Build history of the part. All positions in model axes, mm. A direction names the side the tool comes from. Give positions to 0.01 mm unless a question says otherwise; leave off trailing zeros. Loops run counter-clockwise (first coordinate to the right, second up) from the corner with the lowest first, then second, coordinate; pieces in that order, holes last. Notation, with made-up numbers: M 38,7 L 80,7 A24 ccw 80,33 Z; hole C 53,57.5 d8. An arc over 180 degrees is marked long. Answer in a Markdown table with one row per item. Add a question column.
```python
from build123d import *

# Parameters (mm, degrees)
F0_W          = 120
F0_H          = 13
F0_R          = 1.5
F1_DEPTH      = 13
F2_W          = 120
F2_H          = 5
F3_DEPTH      = 8
F3_DEPTH_BACK = 8
F4_R          = 2.1741492727
F5_DEPTH      = 13
F6_R          = 2
F7_T1_DEPTH   = 16.5
F7_T3_DEPTH   = 16.5
F7_T6_ANGLE   = 90
F7_T8_ANGLE   = 90
F7_T10_ANGLE  = 90
F7_T12_ANGLE  = 90
F7_T14_ANGLE  = 90
F7_T16_ANGLE  = 90
F7_T18_ANGLE  = 90
F7_T20_ANGLE  = 90


# Not quite as in the source:
# - a fillet or chamfer that OpenCascade refuses, or shapes differently, is made with other operations: its cross-section is extruded or revolved along the edge and cut away or added


with BuildPart() as f1:
    # F0 (on Top) → F1 (new body)
    with BuildSketch(Plane.XY):
        Rectangle(F0_W, F0_H)
        with Locations((-55.5, 0)):
            Circle(F0_R, mode=Mode.SUBTRACT)
    extrude(amount=F1_DEPTH)

    # F2 (on Front) → F3 (cut, two sides)
    with BuildSketch(Plane.XZ) as f3_sk:
        with Locations((0, 6.5)):
            Rectangle(F2_W, F2_H)
    extrude(amount=-F3_DEPTH, mode=Mode.SUBTRACT)
    extrude(f3_sk.sketch, amount=F3_DEPTH_BACK, mode=Mode.SUBTRACT)

    # F4 (on Top) → F5 (join)
    with BuildSketch(Plane.XY):
        with Locations((55.0134144723, 0)):
            Circle(F4_R)
    extrude(amount=F5_DEPTH)

    # F6
    f6_edges = [f1.edges().sort_by_distance(p)[0] for p in [
        (0, -6.5, 13),
        (-60, 0, 13),
        (0, 6.5, 13),
        (60, 0, 13),
        (-60, 0, 0),
        (0, -6.5, 0),
        (60, 0, 0),
        (0, 6.5, 0),
    ]]
    fillet(f6_edges, radius=F6_R)

    # F7: fillet of radius 5 on 8 edges, made by hand

    # F7_s2 → F7_t1 (cut)
    with BuildSketch(Plane.XY.offset(-3.5)):
        with BuildLine():
            ThreePointArc((-55, -6.5), (-58.5355339059, -5.0355339059), (-60, -1.5))
            Line((-60, -1.5), (-60, -6.5))
            Line((-60, -6.5), (-55, -6.5))
        make_face()
        with BuildLine():
            ThreePointArc((-55, 6.5), (-58.5355339059, 5.0355339059), (-60, 1.5))
            Line((-60, 1.5), (-60, 6.5))
            Line((-60, 6.5), (-55, 6.5))
        make_face()
        with BuildLine():
            ThreePointArc((60, -1.5), (58.5355339059, -5.0355339059), (55, -6.5))
            Line((55, -6.5), (60, -6.5))
            Line((60, -6.5), (60, -1.5))
        make_face()
        with BuildLine():
            ThreePointArc((60, 1.5), (58.5355339059, 5.0355339059), (55, 6.5))
            Line((55, 6.5), (60, 6.5))
            Line((60, 6.5), (60, 1.5))
        make_face()
    extrude(amount=F7_T1_DEPTH, mode=Mode.SUBTRACT)

    # F7_s4 → F7_t3 (cut)
    with BuildSketch(Plane.XY):
        with BuildLine():
            ThreePointArc((-55, -6.5), (-58.5355339059, -5.0355339059), (-60, -1.5))
            Line((-60, -1.5), (-60, -6.5))
            Line((-60, -6.5), (-55, -6.5))
        make_face()
        with BuildLine():
            ThreePointArc((-55, 6.5), (-58.5355339059, 5.0355339059), (-60, 1.5))
            Line((-60, 1.5), (-60, 6.5))
            Line((-60, 6.5), (-55, 6.5))
        make_face()
        with BuildLine():
            ThreePointArc((60, -1.5), (58.5355339059, -5.0355339059), (55, -6.5))
            Line((55, -6.5), (60, -6.5))
            Line((60, -6.5), (60, -1.5))
        make_face()
        with BuildLine():
            ThreePointArc((60, 1.5), (58.5355339059, 5.0355339059), (55, 6.5))
            Line((55, 6.5), (60, 6.5))
            Line((60, 6.5), (60, 1.5))
        make_face()
    extrude(amount=F7_T3_DEPTH, mode=Mode.SUBTRACT)

    # F7_s5 → F7_t6 (revolve, cut)
    with BuildSketch(Plane.YZ.offset(55)):
        with BuildLine():
            ThreePointArc((4.5, 0), (5.9142135624, 0.5857864376), (6.5, 2))
            Line((6.5, 2), (6.5, 0))
            Line((6.5, 0), (4.5, 0))
        make_face()
    revolve(axis=Axis((55, 1.5, 0), (0, 0, -1)), revolution_arc=F7_T6_ANGLE, mode=Mode.SUBTRACT)

    # F7_s7 → F7_t8 (revolve, cut)
    with BuildSketch(Plane.XZ.offset(1.5)):
        with BuildLine():
            ThreePointArc((58, 0), (59.4142135624, 0.5857864376), (60, 2))
            Line((60, 2), (60, 0))
            Line((60, 0), (58, 0))
        make_face()
    revolve(axis=Axis((55, -1.5, 0), (0, 0, -1)), revolution_arc=F7_T8_ANGLE, mode=Mode.SUBTRACT)

    # F7_s9 → F7_t10 (revolve, cut)
    with BuildSketch(Plane.XZ.offset(-1.5)):
        with BuildLine():
            ThreePointArc((58, 13), (59.4142135624, 12.4142135624), (60, 11))
            Line((60, 11), (60, 13))
            Line((60, 13), (58, 13))
        make_face()
    revolve(axis=Axis((55, 1.5, 13), (0, 0, 1)), revolution_arc=F7_T10_ANGLE, mode=Mode.SUBTRACT)

    # F7_s11 → F7_t12 (revolve, cut)
    with BuildSketch(Plane.YZ.offset(55)):
        with BuildLine():
            ThreePointArc((-4.5, 13), (-5.9142135624, 12.4142135624), (-6.5, 11))
            Line((-6.5, 11), (-6.5, 13))
            Line((-6.5, 13), (-4.5, 13))
        make_face()
    revolve(axis=Axis((55, -1.5, 13), (0, 0, 1)), revolution_arc=F7_T12_ANGLE, mode=Mode.SUBTRACT)

    # F7_s13 → F7_t14 (revolve, cut)
    with BuildSketch(Plane.XZ.offset(-1.5)):
        with BuildLine():
            ThreePointArc((-58, 0), (-59.4142135624, 0.5857864376), (-60, 2))
            Line((-60, 2), (-60, 0))
            Line((-60, 0), (-58, 0))
        make_face()
    revolve(axis=Axis((-55, 1.5, 0), (0, 0, -1)), revolution_arc=F7_T14_ANGLE, mode=Mode.SUBTRACT)

    # F7_s15 → F7_t16 (revolve, cut)
    with BuildSketch(Plane.YZ.offset(-55)):
        with BuildLine():
            ThreePointArc((-4.5, 0), (-5.9142135624, 0.5857864376), (-6.5, 2))
            Line((-6.5, 2), (-6.5, 0))
            Line((-6.5, 0), (-4.5, 0))
        make_face()
    revolve(axis=Axis((-55, -1.5, 0), (0, 0, -1)), revolution_arc=F7_T16_ANGLE, mode=Mode.SUBTRACT)

    # F7_s17 → F7_t18 (revolve, cut)
    with BuildSketch(Plane.YZ.offset(-55)):
        with BuildLine():
            ThreePointArc((4.5, 13), (5.9142135624, 12.4142135624), (6.5, 11))
            Line((6.5, 11), (6.5, 13))
            Line((6.5, 13), (4.5, 13))
        make_face()
    revolve(axis=Axis((-55, 1.5, 13), (0, 0, 1)), revolution_arc=F7_T18_ANGLE, mode=Mode.SUBTRACT)

    # F7_s19 → F7_t20 (revolve, cut)
    with BuildSketch(Plane.XZ.offset(1.5)):
        with BuildLine():
            ThreePointArc((-58, 13), (-59.4142135624, 12.4142135624), (-60, 11))
            Line((-60, 11), (-60, 13))
            Line((-60, 13), (-58, 13))
        make_face()
    revolve(axis=Axis((-55, -1.5, 13), (0, 0, 1)), revolution_arc=F7_T20_ANGLE, mode=Mode.SUBTRACT)


solid = f1.part
```
(1) Wall check: line 1 (Z direction, x = 32.5, y = -1.5); line 2 (Y direction, x = -26, z = 1.75); line 3 (Z direction, x = 49, y = 5.25). Give the ranges that are in metal, low to high.
(2) Slice it at B-B, the plane y = 0. Give the cut face in (x, z), then the cut area to 3 significant figures.
(3) Slice it at A-A, the plane x = -34. Give the cut face in (y, z), then the cut area to 3 significant figures.
(4) Pin check, flat tip, straight feed: pin 1 (1.5 mm diameter, centred on x = -16, z = 7.5, fed in from -Y). Stop position of the tip, or through.
(5) Tool access for faces 5 (the cylindrical face through (58.57, 5, 2.99)), 6 (the cylindrical face through (52.84, 0.1, 6.46)): list every direction of +Z, -Z, +X, -X, +Y, -Y with a clear straight run to the whole face (end or side of a thin tool).
(6) Pull direction Y, two halves, no side cores. Call faces 1 (the cylindrical face through (-54, 0, 11)), 2 (the cylindrical face through (58.57, -5, 9.99)), 3 (the flat face through (-1, 6.5, 3)), 4 (the flat face through (-60, 0, 10)): +Y half, -Y half, draft (parallel to the pull), parting line (faces both ways), or undercut.
Solution:
| question | item | result |
|---|---|---|
| 1 | line 1 | 0 to 4, 9 to 13 |
| 1 | line 2 | -6.48 to 6.48 |
| 1 | line 3 | 0.15 to 4, 9 to 12.85 |
| 2 | outline | M -60,2 A2 ccw -58,0 L -57,0 L -57,4 L -60,4 Z; M -60,9 L -57,9 L -57,13 L -58,13 A2 ccw -60,11 Z; M -54,0 L 58,0 A2 ccw 60,2 L 60,4 L 57.19,4 L 57.19,9 L 60,9 L 60,11 A2 ccw 58,13 L -54,13 L -54,9 L 52.84,9 L 52.84,4 L -54,4 Z |
| 2 | area | 954 mm^2 |
| 3 | outline | M -6.5,2 A2 ccw -4.5,0 L 4.5,0 A2 ccw 6.5,2 L 6.5,4 L -6.5,4 Z; M -6.5,9 L 6.5,9 L 6.5,11 A2 ccw 4.5,13 L -4.5,13 A2 ccw -6.5,11 Z |
| 3 | area | 101 mm^2 |
| 4 | pin 1 | through |
| 5 | face 5 | +Z, -Z, +X, +Y |
| 5 | face 6 | none |
| 6 | face 1 | undercut |
| 6 | face 2 | -Y half |
| 6 | face 3 | +Y half |
| 6 | face 4 | draft |
